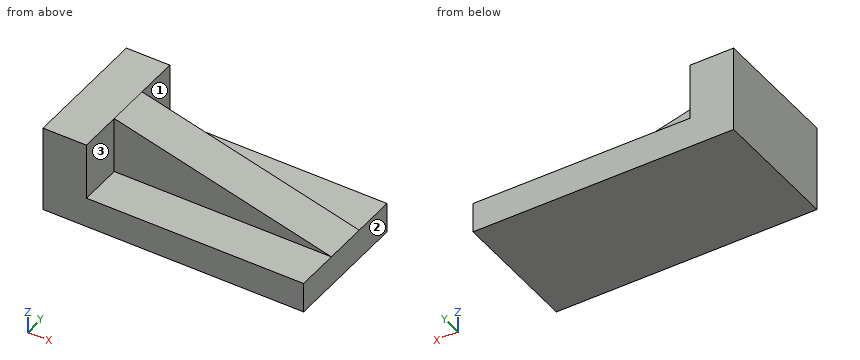
from build123d import *

# Parameters (mm, degrees)
F1_DEPTH = 76.2
F3_DEPTH = 25.4
F5_DEPTH = 25.4


with BuildPart() as f1:
    # F0 (on Front) → F1 (new body)
    with BuildSketch(Plane.XZ):
        Polygon((0, 50.8), (0, 0), (152.4, 0), (152.4, 17.720935), (25.4, 50.8), align=None)
    extrude(amount=-F1_DEPTH)

    # F2 (on face) → F3 (cut)
    with BuildSketch(Plane.XZ):
        Polygon((25.4, 17.720935), (152.4, 17.720935), (25.4, 50.8), align=None)
    extrude(amount=-F3_DEPTH, mode=Mode.SUBTRACT)

    # F4 (on face) → F5 (cut)
    with BuildSketch(Plane(origin=(0, 76.2, 0), x_dir=(-1, 0, 0), z_dir=(0, 1, 0))):
        Polygon((-25.4, 50.8), (-152.4, 17.720935), (-25.4, 17.720935), align=None)
    extrude(amount=-F5_DEPTH, mode=Mode.SUBTRACT)


solid = f1.part
Build history of the part. All positions in model axes, mm. Face numbers are marked on the shaded views. A direction names the side the tool comes from. Round coordinates to 2 decimals unless told otherwise and drop trailing zeros. Write each loop counter-clockwise with the first axis right and the second up, starting at its lowest first coordinate (ties: lowest second). Pieces come first, ordered by that corner, then holes. Notation, with made-up numbers: (-20, -22.75) -> (6, -22.75) arc R25 cw to (6, 1.25) -> close; hole circle Ø2 at (58, 56). An arc over 180 degrees is marked (long way). Write item = value, one per line.
(1) Band-saw the part on B-B (x = 47). Give the cut face in (y, z), then the cut area to 3 significant figures.
Answer:
outline = (0, 0) -> (76.2, 0) -> (76.2, 17.72) -> (50.8, 17.72) -> (50.8, 45.17) -> (25.4, 45.17) -> (25.4, 17.72) -> (0, 17.72) -> close
area = 2,050 mm2
(2) Flat gauge pins, fed straight in: pin 1 (12.5 mm diameter, centred on x = 112, y = 14, fed in from +Z); pin 2 (7.5 mm diameter, centred on y = 59.5, z = 33, fed in from +X); pin 3 (2 mm diameter, centred on x = 72, z = 25.5, fed in from -Y). Where does each tip first touch, or does it go through?
Answer:
pin_1 = 17.72
pin_2 = 25.4
pin_3 = 25.4
(3) Band-saw the part on D-D (y = 67.5). Give the cut face in (x, z), then the cut area to 3 significant figures.
Answer:
outline = (0, 0) -> (152.4, 0) -> (152.4, 17.72) -> (25.4, 17.72) -> (25.4, 50.8) -> (0, 50.8) -> close
area = 3,540 mm2
(4) Band-saw the part on A-A (y = 35). Give the cut face in (x, z).
Answer:
outline = (0, 0) -> (152.4, 0) -> (152.4, 17.72) -> (25.4, 50.8) -> (0, 50.8) -> close
(5) Band-saw the part on C-C (z = 40). Give the cut face in (x, y), then the cut area to 3 significant figures.
Answer:
outline = (0, 0) -> (25.4, 0) -> (25.4, 25.4) -> (66.86, 25.4) -> (66.86, 50.8) -> (25.4, 50.8) -> (25.4, 76.2) -> (0, 76.2) -> close
area = 2,990 mm2
(6) Probe L1, parallel to Y at x = 64, z = 36; L2, parallel to Z at x = 103, y = 10.5; L3, parallel to X at y = 20.5, z = 35.5. List the from-to ranges inside material, lowest first.
Answer:
L1 = 25.4 to 50.8
L2 = 0 to 17.72
L3 = 0 to 25.4
(7) Tool access for the marked faces 1, 2 and 3: list every direction of +Z, -Z, +X, -X, +Y, -Y with a clear straight run to the whole face (end or side of a thin tool).
Answer:
face_1 = +Z, +X, +Y
face_2 = +Z, -Z, +X, +Y, -Y
face_3 = +Z, +X, -Y
